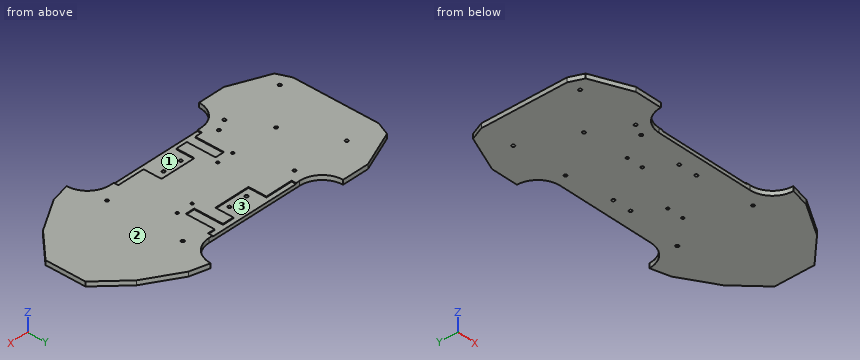
```python
from build123d import *

# Parameters (mm, degrees)
BOSS_EXTRU_1_DEPTH      = 5
D_GAGEMENT_M2_51_D      = 2.9
D_GAGEMENT_M2_51_DEPTH  = 5
D_GAGEMENT_M2_51_TIP    = 0.871247898
D_GAGEMENT_M31_D        = 3.4
D_GAGEMENT_M31_DEPTH    = 6
D_GAGEMENT_M31_TIP      = 1.021463052
D_GAGEMENT_M32_D        = 3.4
D_GAGEMENT_M32_DEPTH    = 5
D_GAGEMENT_M32_TIP      = 1.021463052
ENL_V_MAT_EXTRU_1_DEPTH = 1
ESQUISSE10_3_R          = 1.7
ENL_V_MAT_EXTRU_2_DEPTH = 1
D_GAGEMENT_M33_D        = 3.4
D_GAGEMENT_M33_DEPTH    = 6
D_GAGEMENT_M33_TIP      = 1.021463052
D_GAGEMENT_M34_D        = 3.4
D_GAGEMENT_M34_DEPTH    = 5
D_GAGEMENT_M34_TIP      = 1.021463052


with BuildPart() as part:
    # Esquisse1 → Boss.-Extru.1 (new body)
    with BuildSketch(Plane.XY):
        with BuildLine():
            Line((-87.472008168, 59.584338106), (-117.472008168, 59.584338106))
            Line((-117.472008168, 59.584338106), (-159.472008168, 42.084338106))
            Line((-159.472008168, 42.084338106), (-165.722008168, 27.084338106))
            Line((-165.722008168, 27.084338106), (-165.722008168, -68.315661894))
            Line((-165.722008168, -68.315661894), (-159.472008168, -83.315661894))
            Line((-159.472008168, -83.315661894), (-117.472008168, -100.815661894))
            Line((-117.472008168, -100.815661894), (-87.472008168, -100.815661894))
            ThreePointArc((-87.472008168, -100.815661894), (-80.091099054, -82.996571008), (-62.272008168, -75.615661894))
            Line((-62.272008168, -75.615661894), (47.327991832, -75.615661894))
            ThreePointArc((47.327991832, -75.615661894), (65.147082718, -82.996571008), (72.527991832, -100.815661894))
            Line((72.527991832, -100.815661894), (93.527991832, -95.815661894))
            Line((93.527991832, -95.815661894), (131.527991832, -72.815661894))
            Line((131.527991832, -72.815661894), (161.027991832, -42.815661894))
            Line((161.027991832, -42.815661894), (161.027991832, 1.684338106))
            Line((161.027991832, 1.684338106), (131.527991832, 31.184338106))
            Line((131.527991832, 31.184338106), (93.527991832, 54.184338106))
            Line((93.527991832, 54.184338106), (72.527991832, 59.584338106))
            ThreePointArc((72.527991832, 59.584338106), (65.147082718, 41.76524722), (47.327991832, 34.384338106))
            Line((47.327991832, 34.384338106), (-62.272008168, 34.384338106))
            ThreePointArc((-62.272008168, 34.384338106), (-80.091099054, 41.76524722), (-87.472008168, 59.584338106))
        make_face()
    extrude(amount=BOSS_EXTRU_1_DEPTH)

    # D_gagement M2.51
    with Locations(Plane(origin=(0, 0, 0), x_dir=(-1, 0, 0), z_dir=(0, 0, -1))):
        with Locations((-21.027991832, -8.66564946), (-39.027991832, -8.66564946), (35.972008168, -32.565674331), (53.972008168, -32.565674331)):
            Hole(D_GAGEMENT_M2_51_D / 2, depth=D_GAGEMENT_M2_51_DEPTH)
            with Locations((0, 0, -(D_GAGEMENT_M2_51_DEPTH + D_GAGEMENT_M2_51_TIP / 2))):  # 118° drill point
                Cone(0, D_GAGEMENT_M2_51_D / 2, D_GAGEMENT_M2_51_TIP, mode=Mode.SUBTRACT)

    # D_gagement M31
    with Locations(Plane(origin=(0, 0, 0), x_dir=(-1, 0, 0), z_dir=(0, 0, -1))):
        with Locations((17.896581687, 16.134338106), (-2.752565352, 16.134338106), (18.196581687, -57.365661894), (-2.452565352, -57.365661894)):
            Hole(D_GAGEMENT_M31_D / 2, depth=D_GAGEMENT_M31_DEPTH)
            with Locations((0, 0, -(D_GAGEMENT_M31_DEPTH + D_GAGEMENT_M31_TIP / 2))):  # 118° drill point
                Cone(0, D_GAGEMENT_M31_D / 2, D_GAGEMENT_M31_TIP, mode=Mode.SUBTRACT)

    # D_gagement M32
    with Locations(Plane(origin=(0, 0, 0), x_dir=(-1, 0, 0), z_dir=(0, 0, -1))):
        with Locations((69.972008168, -62.728910548), (69.972008168, 21.49758676), (-65.027991832, -62.728910548), (-65.027991832, 21.49758676)):
            Hole(D_GAGEMENT_M32_D / 2, depth=D_GAGEMENT_M32_DEPTH)
            with Locations((0, 0, -(D_GAGEMENT_M32_DEPTH + D_GAGEMENT_M32_TIP / 2))):  # 118° drill point
                Cone(0, D_GAGEMENT_M32_D / 2, D_GAGEMENT_M32_TIP, mode=Mode.SUBTRACT)

    # Esquisse10 → Enl_v. mat.-Extru.1 (cut)
    with BuildSketch(Plane.XY.offset(5)):
        Polygon((43.027991832, -75.615661894), (43.027991832, -70.615661894), (12.42027445, -70.615661894), (12.42027445, -50.615661894), (-27.372008168, -50.615661894), (-27.372008168, -70.615661894), (-36.072008168, -70.615661894), (-39.872008168, -70.615661894), (-39.872008168, -38.615661894), (-50.072008168, -38.615661894), (-50.072008168, -70.615661894), (-57.972008168, -70.615661894), (-57.972008168, -75.615661894), align=None)
    extrude(amount=-ENL_V_MAT_EXTRU_1_DEPTH, mode=Mode.SUBTRACT)

    # Esquisse10_3 → Enl_v. mat.-Extru.2 (cut)
    with BuildSketch(Plane.XY.offset(5)):
        Polygon((43.027991832, 29.384338106), (43.027991832, 34.384338106), (-57.972008168, 34.384338106), (-57.972008168, 29.384338106), (-27.572008168, 29.384338106), (-27.572008168, 9.384338106), (12.427991832, 9.384338106), (12.427991832, 29.384338106), (24.927991832, 29.384338106), (24.927991832, -2.615661894), (35.127991832, -2.615661894), (35.127991832, 29.384338106), align=None)
        with Locations(Location((-17.896581687, 16.134338106, 0), (0, 0, 180.000000005))):
            Circle(ESQUISSE10_3_R, mode=Mode.SUBTRACT)
        with Locations(Location((2.752565352, 16.134338106, 0), (0, 0, 180.000000005))):
            Circle(ESQUISSE10_3_R, mode=Mode.SUBTRACT)
    extrude(amount=-ENL_V_MAT_EXTRU_2_DEPTH, mode=Mode.SUBTRACT)

    # D_gagement M33
    with Locations(Plane(origin=(0, 0, 0), x_dir=(-1, 0, 0), z_dir=(0, 0, -1))):
        with Locations((104.471408589, -30.715661894), (129.871408589, 24.484338106)):
            Hole(D_GAGEMENT_M33_D / 2, depth=D_GAGEMENT_M33_DEPTH)
            with Locations((0, 0, -(D_GAGEMENT_M33_DEPTH + D_GAGEMENT_M33_TIP / 2))):  # 118° drill point
                Cone(0, D_GAGEMENT_M33_D / 2, D_GAGEMENT_M33_TIP, mode=Mode.SUBTRACT)

    # D_gagement M34
    with Locations(Plane(origin=(0, 0, 0), x_dir=(-1, 0, 0), z_dir=(0, 0, -1))):
        with Locations((150.571408589, -69.115661894), (83.571408589, -69.115661894)):
            Hole(D_GAGEMENT_M34_D / 2, depth=D_GAGEMENT_M34_DEPTH)
            with Locations((0, 0, -(D_GAGEMENT_M34_DEPTH + D_GAGEMENT_M34_TIP / 2))):  # 118° drill point
                Cone(0, D_GAGEMENT_M34_D / 2, D_GAGEMENT_M34_TIP, mode=Mode.SUBTRACT)


solid = part.part
```
Part model, mm, in its own coordinate system. Face numbers are marked on the shaded views. Coordinates: 2 decimals unless noted, no trailing zeros. Order: outer loops, then holes, each group sorted by start corner. A loop starts at its lowest first (then second) coordinate and runs counter-clockwise, first axis right, second up. Notation, with made-up numbers: (11.25, 6) - (24.25, 6) arc R35 cw to (24.25, 42) - close; hole circle Ø8 at (54.25, 61.25). An arc over 180 degrees is marked (long way). Return JSON: item names as keys, results as strings. Group by question number.
Item 1: Cut at A-A (x = -23.5). List the corners of the cut face in (y, z).
Item 2: Cut at D-D (x = -123). List the corners of the cut face in (y, z).
Item 3: Pull direction X, two halves, no side cores. Call the marked faces 1, 2 and 3: pulls with the +X half, pulls with the -X half, needs draft (parallel to the pull), parting line crosses it, or undercut.
Item 4: Cut at B-B (y = 49.5). List the corners of the cut face in (x, z), plus the area to 3 significant figures.
Item 5: Cut at C-C (z = 2.75). State how many separate pieces and enclosed holes the cut face has, plus the area to 3 significant figures.
Item 6: Pin check, flat tips, straight feed: pin 1 (1 mm diameter, centred on x = -48, z = 1, fed in from +Y); pin 2 (3 mm diameter, centred on y = -68, z = 3, fed in from +X); pin 3 (4.5 mm diameter, centred on x = -18.2, y = -57.37, fed in from +Z). Stop position of each tip, or through.
Item 7: Drill centre lines: probe 1 along Y at (x, z) = (-69, 3.6); probe 2 along Y at (x, z) = (-69.5, 3); probe 3 along X at (y, z) = (-9.5, 3.8). Where is each one in solid material? Low to high. Write a range as from..to.
Check values:
{
 "1": {"outline": "(-75.62, 0) - (34.38, 0) - (34.38, 4) - (9.38, 4) - (9.38, 5) - (-50.62, 5) - (-50.62, 4) - (-75.62, 4) - close"},
 "2": {"outline": "(-98.51, 0) - (57.28, 0) - (57.28, 5) - (-98.51, 5) - close"},
 "3": {"face 1": "undercut", "face 2": "needs draft", "face 3": "undercut"},
 "4": {"outline": "(-141.67, 0) - (-85.37, 0) - (-85.37, 5) - (-141.67, 5) - close; (70.42, 0) - (101.27, 0) - (101.27, 5) - (70.42, 5) - close", "area": "436 mm2"},
 "5": {"separate pieces": "1", "enclosed holes": "16", "area": "39,800 mm2"},
 "6": {"pin 1": "stops at y = 34.38", "pin 2": "stops at x = 137.74", "pin 3": "stops at z = 4"},
 "7": {"probe 1": "y = -76.53..-64.12, -61.33..20.1, 22.89..35.3", "probe 2": "y = -76.67..-64.36, -61.1..19.86, 23.13..35.44", "probe 3": "x = -165.72..19.84, 22.21..37.84, 40.21..161.03"}
}
